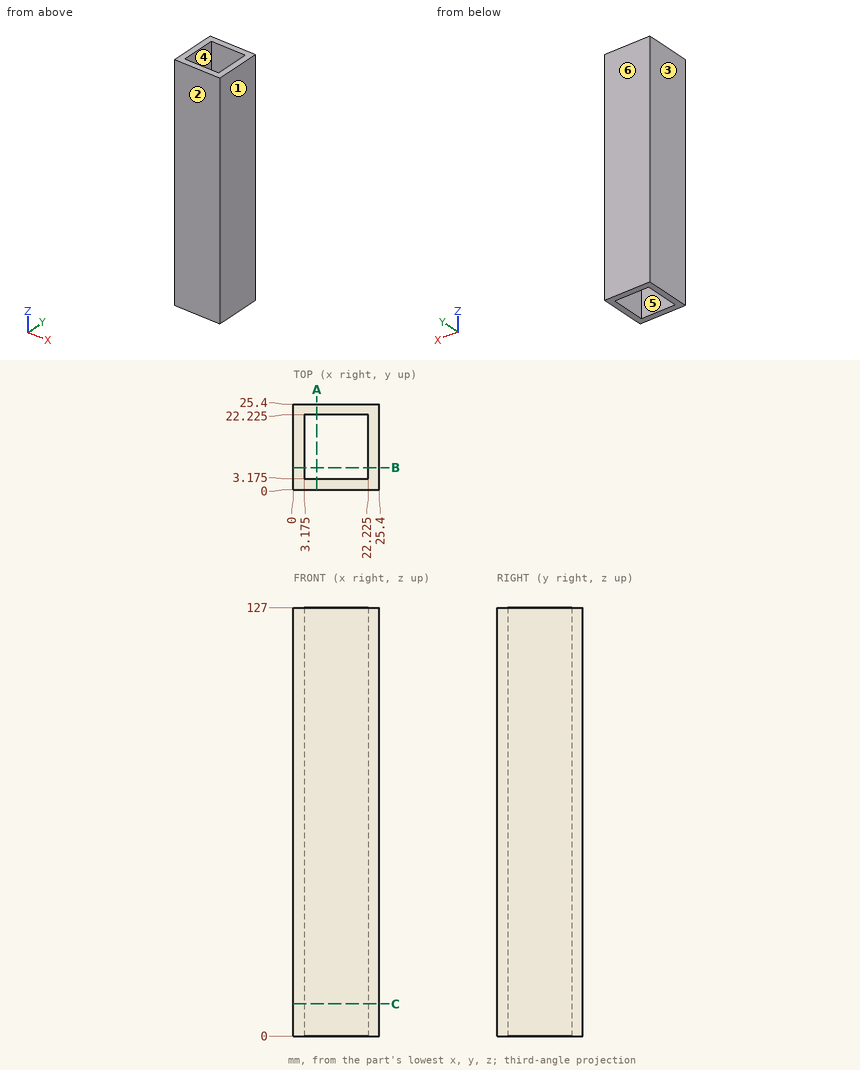
For this review, use the dimensioned drawing (mm, ordinates from the lowest corner) and the shaded views. A direction names the side the tool comes from. Round coordinates to 2 decimals unless told otherwise and drop trailing zeros. Order: outer loops, then holes, each group sorted by start corner. A loop starts at its lowest first (then second) coordinate and runs counter-clockwise, first axis right, second up. Notation, with made-up numbers: (46, 43) -> (66, 43) arc R20 ccw to (66, 64) -> close; hole circle Ø6 at (31.5, 44). An arc over 180 degrees is marked (long way). Put each result on its own line as item: value.
Q1. Mouldability with a two-part tool opening along X and no side actions: class the marked faces 1, 2, 3 and 4 as pulls with the +X half, pulls with the -X half, needs draft (parallel to the pull), parting line crosses it, or undercut.
Check result:
face 1: pulls with the +X half
face 2: needs draft
face 3: pulls with the -X half
face 4: undercut
Q2. For probe 1 along X at (y, z) = (21.5, 106.5) (3 decimals), list the stretches that pass through material, from the lowest coordinate up. Write a range as [from, to].
Check result:
probe 1: [0, 3.175], [22.225, 25.4]
Q3. Add section C-C on z = 9.5. Write out the cut boundary in (x, y) (3 decimals), plus the area to 3 significant figures.
Check result:
outline: (0, 0) -> (25.4, 0) -> (25.4, 25.4) -> (0, 25.4) -> close; hole (3.175, 3.175) -> (22.225, 3.175) -> (22.225, 22.225) -> (3.175, 22.225) -> close
area: 282 mm2
Q4. Machinability: for the marked faces 5 and 6, which of the approach directions +Z, -Z, +X, -X, +Y, -Y give a long, thin tool a straight path to every point of the face, cutting with its end or side? Answer none if there is none.
Check result:
face 5: +Z, -Z
face 6: +Z, -Z, +X, -X, +Y
Q5. Add section A-A on x = 7. Write out the cut boundary in (y, z) (3 decimals), plus the area to 3 significant figures.
Check result:
outline: (0, 0) -> (3.175, 0) -> (3.175, 127) -> (0, 127) -> close; (22.225, 0) -> (25.4, 0) -> (25.4, 127) -> (22.225, 127) -> close
area: 806 mm2
